Work out the finished part from the listing and answer in its coordinate system (mm). A direction names the side the tool comes from. Coordinates: 2 decimals unless noted, no trailing zeros. Write each loop counter-clockwise with the first axis right and the second up, starting at its lowest first coordinate (ties: lowest second). Pieces come first, ordered by that corner, then holes. Notation, with made-up numbers: M 40.5,-15.75 L 53.5,-15.75 A13 cw 53.5,9.25 Z; hole C 0.5,29.25 d4. An arc over 180 degrees is marked long. Use CSV: the item, a comma, the result in double quotes.
from build123d import *

# Parameters (mm, degrees)
SKETCH4_R           = 8.5
BOSS_EXTRUDE1_DEPTH = 5


with BuildPart() as part:
    # Sketch4 → Boss-Extrude1 (new body)
    with BuildSketch(Plane(origin=(0, 0, 0), x_dir=(0, 1, 0), z_dir=(0, 0, 1))):
        Polygon((-40, -30), (-30.267949192, -30), (-32, -27), (-22.90673326, -27), (-13.813466521, -27), (-15.545517328, -30), (-7.361215932, -30), (-9.09326674, -27), (3.1e-08, -27), (9.09326674, -27), (7.361215932, -30), (15.545517328, -30), (13.813466521, -27), (22.90673326, -27), (32, -27), (30.267949192, -30), (40, -30), (40, -7.447818473), (37, -9.17986928), (37, -5.1e-08), (37, 9.17986928), (40, 7.447818473), (40, 30), (30.267949192, 30), (32, 27), (22.90673326, 27), (13.813466521, 27), (15.545517328, 30), (7.361215932, 30), (9.09326674, 27), (0, 27), (-9.09326674, 27), (-7.361215932, 30), (-15.545517328, 30), (-13.813466521, 27), (-22.90673326, 27), (-32, 27), (-30.267949192, 30), (-40, 30), (-40, 7.447818473), (-37, 9.17986928), (-37, 0), (-37, -9.17986928), (-40, -7.447818473), align=None)
        with Locations(Location((0, 0, 0), (0, 0, 270))):
            Circle(SKETCH4_R, mode=Mode.SUBTRACT)
    extrude(amount=BOSS_EXTRUDE1_DEPTH)


solid = part.part
Item 1: For a pull along Y with two mould halves and no side action, classify faces 1 (the face through (-30, 12, 2)), 2 (the face through (19, 40, 2)), 3 (the face through (28.521, -8.215, 2.465)) as released by +Y, released by -Y, zero draft, split by the parting line, or undercut.
Answer:
face 1,"zero draft"
face 2,"released by +Y"
face 3,"undercut"
Item 2: A tool of negligible diameter and unlimited length cuts with its end or side. For faces 4 (the face through (0, -9, 0)), 5 (the face through (-27, 23, 2)), from which of +Z, -Z, +X, -X, +Y, -Y can it reach the whole face along a straight path? Write none if from no direction.
Answer:
face 4,"-Z, +X, -X, +Y, -Y"
face 5,"+Z, -Z"
Item 3: The part is cut by section A-A (y = 0). Write down the section's boundary in (x, z), then the cut area to 3 significant figures.
Answer:
outline,"M -27,0 L -8.5,0 L -8.5,5 L -27,5 Z; M 8.5,0 L 27,0 L 27,5 L 8.5,5 Z"
area,"185 mm2"
Item 4: Given pin 1 (1 mm diameter, centred on y = -21, z = 1.5, fed in from +X); pin 2 (1.5 mm diameter, centred on y = -23, z = 1.5, fed in from -X); pin 3 (1.5 mm diameter, centred on x = -2.5, z = 2, fed in from +Y), each flat-ended and moving along its own axis, determine where each tip first touches the part or whether it passes through.
Answer:
pin 1,"stops at x = 27"
pin 2,"stops at x = -27"
pin 3,"stops at y = 37"
Item 5: The part is cut by section B-B (x = 0). Write down the section's boundary in (y, z), then the cut area to 3 significant figures.
Answer:
outline,"M -37,0 L -8.5,0 L -8.5,5 L -37,5 Z; M 8.5,0 L 37,0 L 37,5 L 8.5,5 Z"
area,"285 mm2"
Item 6: Consider probe 1 along Y at (x, z) = (0, 1.2); probe 2 along X at (y, z) = (-16, 1.4); probe 3 along X at (y, z) = (14, 0.95). Determine where each line is inside the solid, lowest interval first.
Answer:
probe 1,"y = -37 to -8.5, 8.5 to 37"
probe 2,"x = -27 to 27"
probe 3,"x = -30 to -27.32, -27 to 27, 27.32 to 30"
